```python
from build123d import *

# Parameters (mm, degrees)
F1_DEPTH = 101.6
F2_DEPTH = 50.8
F3_DEPTH = 50.8
F5_DEPTH = 12.7


with BuildPart() as f1:
    # F0 (on Front) → F1 (new body)
    with BuildSketch(Plane.XZ):
        Polygon((0, 61.214138), (0, 0), (3.565873, 0), (3.565873, 2.286), (3.565873, 57.973351), (3.565873, 61.214138), align=None)
    extrude(amount=F1_DEPTH)

    # F0 (on Front) → F2 (join)
    with BuildSketch(Plane.XZ):
        Polygon((3.565873, 2.286), (3.565873, 0), (64.482857, 0), (3.565873, 61.214138), (3.565873, 57.973351), (58.982899, 2.286), align=None)
    extrude(amount=F2_DEPTH)

    # F0 (on Front) → F3 (join)
    with BuildSketch(Plane.XZ):
        Polygon((0, 61.214138), (0, 0), (3.565873, 0), (3.565873, 2.286), (3.565873, 57.973351), (3.565873, 61.214138), align=None)
    extrude(amount=-F3_DEPTH)

    # F4 (on Top) → F5 (join)
    with BuildSketch(Plane.XY):
        Polygon((0, 47.907468), (0, 50.730321), (-63.773681, -25.40238), (0, -101.535082), (0, -98.203303), (-61.195922, -25.147918), align=None)
    extrude(amount=F5_DEPTH)


solid = f1.part
```
Check sheet for the modelled part. Datum: model origin and axes. Units: mm. A direction names the side the tool comes from. Round coordinates to 2 decimals unless told otherwise and drop trailing zeros. Order: outer loops, then holes, each group sorted by start corner. A loop starts at its lowest first (then second) coordinate and runs counter-clockwise, first axis right, second up. Notation, with made-up numbers: M -38,47.25 L 19,47.25 A19 ccw 19,68.25 Z; hole C 77.25,61.25 d6. An arc over 180 degrees is marked long. Answer in a Markdown table with one row per item.
(1) Section check A-A on y = -38.5. Record the boundary of the cut face in (x, z).
Findings:
| item | result |
|---|---|
| outline | M -52.8,0 L -50.01,0 L -50.01,12.7 L -52.8,12.7 Z; M 0,0 L 64.48,0 L 3.57,61.21 L 0,61.21 Z; hole M 3.57,2.29 L 58.98,2.29 L 3.57,57.97 Z |
(2) Draft check along Y on faces 1 (the flat face through (-30.17, -62.187, 6.261)), 2 (the flat face through (38, 0, 24)), 3 (the flat face through (32, -25, 2.286)), 4 (the flat face through (-31, 10.9, 6.3)). Enter one of: +Y half, -Y half, draft (parallel to the pull), parting line (faces both ways), or undercut.
Findings:
| item | result |
|---|---|
| face 1 | undercut |
| face 2 | +Y half |
| face 3 | draft |
| face 4 | undercut |
(3) Section check C-C on x = 9. Record the boundary of the cut face in (y, z), plus the area to 3 significant figures.
Findings:
| item | result |
|---|---|
| outline | M -50.8,0 L 0,0 L 0,2.29 L -50.8,2.29 Z; M -50.8,52.51 L 0,52.51 L 0,55.75 L -50.8,55.75 Z |
| area | 281 mm^2 |
(4) Section check D-D on z = 24.5. Record the boundary of the cut face in (x, y), plus the area to 3 significant figures.
Findings:
| item | result |
|---|---|
| outline | M 0,-101.6 L 3.57,-101.6 L 3.57,50.8 L 0,50.8 Z; M 36.88,-50.8 L 40.1,-50.8 L 40.1,0 L 36.88,0 Z |
| area | 707 mm^2 |
(5) Set-up check for faces 5 (the flat face through (-49, -8, 12.7)), 6 (the flat face through (30.886, -25.044, 30.519)), 7 (the flat face through (38, -50.8, 24)), 8 (the flat face through (34.45, -25.04, 30.18)): record each of +Z, -Z, +X, -X, +Y, -Y from which the full face is reachable in a straight line by a thin tool's end or side.
Findings:
| item | result |
|---|---|
| face 5 | +Z, -X, +Y, -Y |
| face 6 | +Y, -Y |
| face 7 | +Z, -Z, +X, -Y |
| face 8 | +Z, +X, +Y, -Y |
(6) Material ranges on line 1 along X through (y, z) = (-90.5, 15); line 2 along X through (y, z) = (-50, 13); line 3 along X through (y, z) = (23, 12.5), recorded low to high. Write a range as from..to.
Findings:
| item | result |
|---|---|
| line 1 | x = 0..3.57 |
| line 2 | x = 0..3.57, 48.32..51.55 |
| line 3 | x = -23.23..-20.86, 0..3.57 |
(7) Section check B-B on z = 6. Record the boundary of the cut face in (x, y), plus the area to 3 significant figures.
Findings:
| item | result |
|---|---|
| outline | M -63.77,-25.4 L 0,-101.54 L 0,-101.6 L 3.57,-101.6 L 3.57,50.8 L 0,50.8 L 0,50.73 Z; M 55.29,-50.8 L 58.51,-50.8 L 58.51,0 L 55.29,0 Z; hole M -61.2,-25.15 L 0,-98.2 L 0,47.91 Z |
| area | 1,090 mm^2 |
(8) Gauge pin test, flat ends, axial feed: pin 1 (18.5 mm diameter, centred on y = -46, z = 44.5, fed in from +X); pin 2 (1.5 mm diameter, centred on x = 51, y = 1, fed in from +Z); pin 3 (10 mm diameter, centred on y = -8, z = 50.5, fed in from -X); pin 4 (1 mm diameter, centred on x = -51, z = 9.5, fed in from -Y). Record the tip position at first contact, or that the pin passes through.
Findings:
| item | result |
|---|---|
| pin 1 | stops at x = 29.4 |
| pin 2 | passes through |
| pin 3 | stops at x = 0 |
| pin 4 | stops at y = -41.25 |
